```python
from build123d import *
from build123d.topology import SkipClean

# Parameters (mm, degrees)
SKETCH1_R           = 27.5
BOSS_EXTRUDE1_DEPTH = 2.5
SKETCH2_R           = 7.1
BOSS_EXTRUDE2_DEPTH = 10
BOSS_EXTRUDE3_DEPTH = 10
CHAMFER1_SIZE       = 1.8
FILLET2_R           = 3


with BuildPart() as part:
    # Sketch1 → Boss-Extrude1 (new body)
    with BuildSketch(Plane(origin=(0, 0, 0), x_dir=(1, 0, 0), z_dir=(0, 1, 0))):
        with Locations(Location((0, 0, 0), (0, 0, 270))):
            Circle(SKETCH1_R)
    extrude(amount=BOSS_EXTRUDE1_DEPTH)

    # Sketch2 → Boss-Extrude2 (add)
    with BuildSketch(Plane(origin=(0, 2.5, 0), x_dir=(1, 0, 0), z_dir=(0, 1, 0))):
        with Locations(Location((0, 0, 0), (0, 0, 270))):
            Circle(SKETCH2_R)
    extrude(amount=BOSS_EXTRUDE2_DEPTH)

    # Sketch5 → Boss-Extrude3 (add)
    with SkipClean():  # the faces are left unmerged after this step: merging them gives an invalid solid
        with BuildSketch(Plane(origin=(0, 2.5, 0), x_dir=(1, 0, 0), z_dir=(0, 1, 0))):
            with BuildLine():
                Line((0, 24.57), (0, 27.5))
                ThreePointArc((0, 27.5), (25.957349719, 9.081078988), (17.143326771, -21.502473049))
                Line((17.143326771, -21.502473049), (15.316783228, -19.211482284))
                ThreePointArc((15.316783228, -19.211482284), (23.191712094, 8.113531299), (0, 24.57))
            make_face()
        extrude(amount=BOSS_EXTRUDE3_DEPTH)

    # Chamfer1
    # the kernel refuses this chamfer: 1.8 mm, written as the material it takes off along each edge
    with BuildSketch(Plane(origin=(0, 2.5, -24.57), x_dir=(0, 0, -1), z_dir=(0, 1, 0))) as chamfer1_piece_1:
        with BuildLine():
            Line((CHAMFER1_SIZE, 0), (-0.071369946, -1.871369946))
            ThreePointArc((-0.071369946, -1.871369946), (-0.018871327, -0.96279846), (0, 0))
            Line((0, 0), (CHAMFER1_SIZE, 0))
        make_face()
    extrude(amount=14.815417609, mode=Mode.SUBTRACT)
    with BuildSketch(Plane(origin=(15.316783228, 2.5, 19.211482284), x_dir=(0.7575824934147944, 0, -0.652739431681144), z_dir=(0, 1, 0))) as chamfer1_piece_2:
        with BuildLine():
            Line((1.872730398, 0), (-CHAMFER1_SIZE * 0.0381101017104, -CHAMFER1_SIZE * 0.999273546206))
            Line((-CHAMFER1_SIZE * 0.0381101017104, -CHAMFER1_SIZE * 0.999273546206), (0, 0))
            ThreePointArc((0, 0), (0.962818219, -0.01783473), (1.872730398, 0))
        make_face()
    extrude(amount=14.815417609, mode=Mode.SUBTRACT)

    # Fillet2
    fillet2_edges = [part.edges().sort_by_distance(p)[0] for p in [
        (1.871369946, 7.5, -24.498630054),
        (16.735530992, 7.5, 17.989077308),
    ]]
    fillet(fillet2_edges, radius=FILLET2_R)


solid = part.part
```
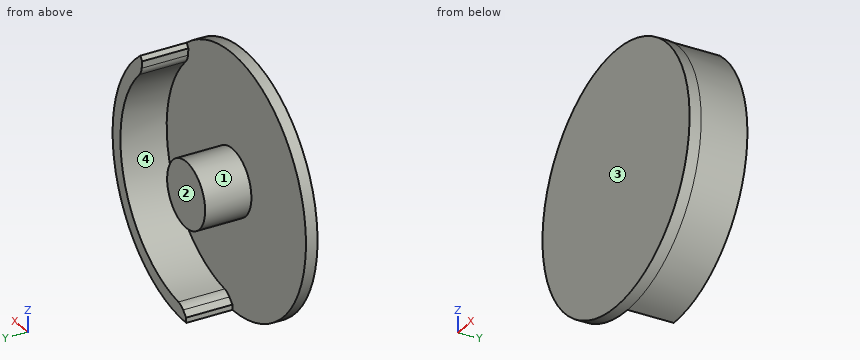
The listing builds one solid part. Answer for the finished solid, in the listing's coordinates (mm). Face numbers are marked on the shaded views. A direction names the side the tool comes from. Coordinates: 2 decimals unless noted, no trailing zeros. Write each loop counter-clockwise with the first axis right and the second up, starting at its lowest first coordinate (ties: lowest second). Pieces come first, ordered by that corner, then holes. Notation, with made-up numbers: (66, 62) - (86, 62) arc R17 cw to (86, 70) - close; hole circle Ø11 at (65, 32.25). An arc over 180 degrees is marked (long way). Return JSON: item names as keys, results as strings. Group by question number.
Q1. The part is cut by section B-B on z = 0. Write down the section's boundary in (x, y).
Q2. The part is cut by section C-C on x = 19.5. Write down the section's boundary in (y, z).
Q3. Flat-ended cylindrical pins translate along their axes: pin 1 Ø2 at (x, z) = (0, 6.5) entering from -Y; pin 2 Ø1.5 at (y, z) = (8, 15) entering from +X; pin 3 Ø6 at (x, y) = (7.5, 10.5) entering from +Z; pin 4 Ø1.2 at (y, z) = (9.5, -27) entering from -X. Find the tip coordinate at first contact, or state that the pin passes through.
Q4. Which of the six approach directions +Z, -Z, +X, -X, +Y, -Y give full straight-line access (tool end or side, diameter ignored) to the marked faces 3 and 4?
Q5. The part is cut by section D-D on z = 9.5. Write down the section's boundary in (x, y), and give its area (3 significant figures).
Q6. Find the intervals of material crossed by line 1 along Y through (x, z) = (-4, -7); line 2 along X through (y, z) = (5.5, 6); line 3 along Z through (x, y) = (3.5, 10), in increasing order. Write a range as [from, to].
Q7. For a pull along Z with two mould halves and no side action, classify the marked faces 1 and 2 as +Z half, -Z half, draft (parallel to the pull), parting line (faces both ways), or undercut.
Q8. The part is cut by section A-A on y = 6.5. Write down the section's boundary in (x, z), and give its area (3 significant figures).
Evaluation:
{
 "1": {"outline": "(-27.5, 0) - (27.5, 0) - (27.5, 12.5) - (24.57, 12.5) - (24.57, 2.5) - (7.1, 2.5) - (7.1, 12.5) - (-7.1, 12.5) - (-7.1, 2.5) - (-27.5, 2.5) - close"},
 "2": {"outline": "(0, -19.39) - (12.5, -19.39) - (12.5, -14.95) - (2.5, -14.95) - (2.5, 14.95) - (12.5, 14.95) - (12.5, 19.39) - (0, 19.39) - close"},
 "3": {"pin 1": "stops at y = 0", "pin 2": "stops at x = 23.52", "pin 3": "stops at z = 5.49", "pin 4": "stops at x = 0"},
 "4": {"face 3": "+Z, -Z, +X, -X, -Y", "face 4": "+Y"},
 "5": {"outline": "(-25.81, 0) - (25.81, 0) - (25.81, 12.5) - (22.66, 12.5) - (22.66, 2.5) - (-25.81, 2.5) - close", "area": "161 mm2"},
 "6": {"line 1": "y = [0, 2.5]", "line 2": "x = [-3.8, 3.8], [23.83, 26.84]", "line 3": "z = [-27.28, -24.32], [-6.18, 6.18]"},
 "7": {"face 1": "undercut", "face 2": "draft"},
 "8": {"outline": "circle Ø14.2 at (0, 0); (0, -27.5) arc R27.5 ccw to (17.14, 21.5) - (16.44, 20.62) - (16.62, 19.06) arc R3 ccw to (17.46, 17.28) arc R24.57 cw to (2.88, -24.4) arc R3 ccw to (1.11, -25.26) - (0, -26.37) - close", "area": "343 mm2"}
}
